Verification items for the finished model (mm, model axes). A direction names the side the tool comes from. Round coordinates to 2 decimals unless told otherwise and drop trailing zeros. Order: outer loops, then holes, each group sorted by start corner. A loop starts at its lowest first (then second) coordinate and runs counter-clockwise, first axis right, second up. Notation, with made-up numbers: (24.5, -31.5) -> (48.5, -31.5) arc R25 ccw to (48.5, -18.5) -> close; hole circle Ø6 at (26.5, 51.5). An arc over 180 degrees is marked (long way). Put each result on its own line as item: value.
from build123d import *

# Parameters (mm, degrees)
BASE_FLANGE1_DEPTH      = 13
BASE_FLANGE1_DEPTH_BACK = 22
SKETCH5_R               = 4
SKETCH5_R_2             = 1.05
CUT_EXTRUDE1_DEPTH      = 10
CUT_EXTRUDE2_DEPTH      = 30.864025181
CUT_EXTRUDE2_DEPTH_BACK = 30.864025181
SKETCH7_R               = 1.3
FILLET1_R               = 2
SKETCH8_R               = 1.3
CUT_EXTRUDE3_DEPTH      = 10
SKETCH9_W               = 12
SKETCH9_H               = 6
CUT_EXTRUDE4_DEPTH      = 10
FILLET2_R               = 1


# Sheet-metal steps are written as plain solids
with BuildPart() as part:
    # Sketch1 → Base-Flange1 (new, two sides: drawn at the far end of the back side and taken through both)
    with BuildSketch(Plane.XY.offset(-BASE_FLANGE1_DEPTH_BACK)):
        with BuildLine():
            Line((-17, 8.1), (-17, 2.5))
            ThreePointArc((-17, 2.5), (-16.267766953, 0.732233047), (-14.5, 0))
            Line((-14.5, 0), (14.5, 0))
            ThreePointArc((14.5, 0), (16.267766953, 0.732233047), (17, 2.5))
            Line((17, 2.5), (17, 8.1))
            Line((17, 8.1), (18.5, 8.1))
            Line((18.5, 8.1), (18.5, 2.5))
            ThreePointArc((18.5, 2.5), (17.328427125, -0.328427125), (14.5, -1.5))
            Line((14.5, -1.5), (-14.5, -1.5))
            ThreePointArc((-14.5, -1.5), (-17.328427125, -0.328427125), (-18.5, 2.5))
            Line((-18.5, 2.5), (-18.5, 8.1))
            Line((-18.5, 8.1), (-17, 8.1))
        make_face()
    extrude(amount=BASE_FLANGE1_DEPTH + BASE_FLANGE1_DEPTH_BACK)

    # Sketch5 → Cut-Extrude1 (cut)
    with BuildSketch(Plane(origin=(0, 0, 0), x_dir=(1, 0, 0), z_dir=(0, 1, 0))):
        with Locations(Location((0, 0, 0), (0, 0, 180))):
            Circle(SKETCH5_R)
        with Locations(Location((0, 8, 0), (0, 0, 180))):
            Circle(SKETCH5_R_2)
        with Locations(Location((5.656854249, 5.656854249, 0), (0, 0, 180))):
            Circle(SKETCH5_R_2)
        with Locations(Location((8, 0, 0), (0, 0, 180))):
            Circle(SKETCH5_R_2)
        with Locations(Location((5.656854249, -5.656854249, 0), (0, 0, 180))):
            Circle(SKETCH5_R_2)
        with Locations(Location((0, -8, 0), (0, 0, 180))):
            Circle(SKETCH5_R_2)
        with Locations(Location((-5.656854249, -5.656854249, 0), (0, 0, 180))):
            Circle(SKETCH5_R_2)
        with Locations(Location((-8, 0, 0), (0, 0, 180))):
            Circle(SKETCH5_R_2)
        with Locations(Location((-5.656854249, 5.656854249, 0), (0, 0, 180))):
            Circle(SKETCH5_R_2)
    extrude(amount=-CUT_EXTRUDE1_DEPTH, mode=Mode.SUBTRACT)

    # Sketch7 → Cut-Extrude2 (cut, two sides: drawn at the far end of the back side and taken through both)
    with BuildSketch(Plane(origin=(0, 0, 0), x_dir=(0, 0, -1), z_dir=(1, 0, 0)).offset(-CUT_EXTRUDE2_DEPTH_BACK)):
        with Locations((-4, 5.5)):
            Circle(SKETCH7_R)
        with Locations((18, 5.5)):
            Circle(SKETCH7_R)
    extrude(amount=CUT_EXTRUDE2_DEPTH + CUT_EXTRUDE2_DEPTH_BACK, mode=Mode.SUBTRACT)

    # Fillet1
    fillet1_edges = [part.edges().sort_by_distance(p)[0] for p in [
        (-17.75, 8.1, 13),
        (-17.75, 8.1, -22),
        (17.75, 8.1, -22),
        (17.75, 8.1, 13),
    ]]
    fillet(fillet1_edges, radius=FILLET1_R)

    # Sketch8 → Cut-Extrude3 (cut)
    with BuildSketch(Plane.XZ.offset(1.5)):
        with Locations(Location((-10, 3, 0), (0, 0, 270))):
            Circle(SKETCH8_R)
        with Locations(Location((10, 3, 0), (0, 0, 270))):
            Circle(SKETCH8_R)
        with Locations(Location((10, -17, 0), (0, 0, 270))):
            Circle(SKETCH8_R)
        with Locations(Location((-10, -17, 0), (0, 0, 270))):
            Circle(SKETCH8_R)
    extrude(amount=-CUT_EXTRUDE3_DEPTH, mode=Mode.SUBTRACT)

    # Sketch9 → Cut-Extrude4 (cut)
    with BuildSketch(Plane.XZ.offset(1.5)):
        with Locations((0, -15)):
            Rectangle(SKETCH9_W, SKETCH9_H)
    extrude(amount=-CUT_EXTRUDE4_DEPTH, mode=Mode.SUBTRACT)

    # Fillet2
    fillet2_edges = [part.edges().sort_by_distance(p)[0] for p in [
        (6, -0.75, -12),
        (6, -0.75, -18),
        (-6, -0.75, -18),
        (-6, -0.75, -12),
    ]]
    fillet(fillet2_edges, radius=FILLET2_R)


solid = part.part
Item 1: Section check A-A on y = 5.5. Record the boundary of the cut face in (x, z), then the cut area to 3 significant figures.
Check sheet entries:
outline: (-18.5, -22) -> (-17, -22) -> (-17, -19.3) -> (-18.5, -19.3) -> close; (-18.5, -16.7) -> (-17, -16.7) -> (-17, 2.7) -> (-18.5, 2.7) -> close; (-18.5, 5.3) -> (-17, 5.3) -> (-17, 13) -> (-18.5, 13) -> close; (17, -22) -> (18.5, -22) -> (18.5, -19.3) -> (17, -19.3) -> close; (17, -16.7) -> (18.5, -16.7) -> (18.5, 2.7) -> (17, 2.7) -> close; (17, 5.3) -> (18.5, 5.3) -> (18.5, 13) -> (17, 13) -> close
area: 89.4 mm^2
Item 2: Section check C-C on z = 3.5. State how many separate pieces and enclosed holes the cut face has, then the cut area to 3 significant figures.
Check sheet entries:
separate pieces: 6
enclosed holes: 0
area: 55.4 mm^2
Item 3: Release check for a two-part mould opening along X. For faces 1 (the cylindrical face through (-8.71, -0.76, 3.17)), 2 (the flat face through (0.1, -0.2, 13)) record: +X half, -X half, draft (parallel to the pull), parting line (faces both ways), or undercut.
Check sheet entries:
face 1: undercut
face 2: draft
Item 4: Gauge pin test, flat ends, axial feed: pin 1 Ø1.7 at (x, z) = (-8, 0) entering from -Y; pin 2 Ø1 at (x, z) = (11.5, 8) entering from +Y; pin 3 Ø0.8 at (y, z) = (-0.5, -15) entering from +X. Record the tip position at first contact, or that the pin passes through.
Check sheet entries:
pin 1: passes through
pin 2: stops at y = 0
pin 3: stops at x = 17.54
Item 5: Material ranges on L1, parallel to X at y = 3.5, z = -3; L2, parallel to Y at x = 5, z = 9.5; L3, parallel to Z at x = 8, y = -0.75, recorded low to high. Write a range as [from, to].
Check sheet entries:
L1: x = [-18.5, -17], [17, 18.5]
L2: y = [-1.5, 0]
L3: z = [-22, -1.05], [1.05, 13]
Item 6: Tool access check on faces 3 (the cylindrical face through (-16.287, 0.752, -4.745)), 4 (the cylindrical face through (5.699, -0.74, -12.285)), 5 (the flat face through (0, -1.5, -5)). Record the directions out of +Z, -Z, +X, -X, +Y, -Y that give a thin tool (end or side, any length) a straight path to the whole face; none if there is none.
Check sheet entries:
face 3: +Z, -Z, +Y
face 4: +Y, -Y
face 5: +Z, -Z, +X, -X, -Y
Item 7: Section check B-B on x = -8. Record the boundary of the cut face in (y, z).
Check sheet entries:
outline: (-1.5, -22) -> (0, -22) -> (0, -1.05) -> (-1.5, -1.05) -> close; (-1.5, 1.05) -> (0, 1.05) -> (0, 13) -> (-1.5, 13) -> close
